The listing builds one solid part. Answer for the finished solid, in the listing's coordinates (mm). A direction names the side the tool comes from. Coordinates: 2 decimals unless noted, no trailing zeros. Order: outer loops, then holes, each group sorted by start corner. A loop starts at its lowest first (then second) coordinate and runs counter-clockwise, first axis right, second up. Notation, with made-up numbers: (-24.5, -2.75) - (-5.5, -2.75) arc R21 cw to (-5.5, 26.25) - close; hole circle Ø11 at (48.5, 71.25). An arc over 180 degrees is marked (long way). Use one line per item in the form item = value. Start each with the question number.
Item 1: The mould has two halves that part along X. Classify faces 1 (the flat face through (-52, 1.5, -61)), 2 (the cylindrical face through (-1.271, 0.021, -129.994)), 3 (the flat face through (48.734, 0.021, -39.41)), 4 (the flat face through (-50.12, 0.02, -41.06)): released by +X, released by -X, zero draft, split by the parting line, or undercut.
Item 2: Section A-A, the plane z = -65.5 is taken. Write down the section's boundary in (x, y).
Item 3: A tool of negligible diameter and unlimited length cuts with its end or side. For faces 5 (the flat face through (-52, -1.5, -61)), 6 (the flat face through (42.366, 0.021, -50.49)), from which of +Z, -Z, +X, -X, +Y, -Y can it reach the whole face along a straight path? Write none if from no direction.
Item 4: Section B-B, the plane x = 55 is taken. Write down the section's boundary in (y, z), and give its area (3 significant figures).
Item 5: Each of these flat-tipped pins is pushed along its axis until it touches: pin 1 Ø1 at (y, z) = (-1, -69.5) entering from +X; pin 2 Ø12 at (x, z) = (7.5, -14.5) entering from -Y; pin 3 Ø2.5 at (x, z) = (-20.65, -11.93) entering from +Y. Where does it stop, or does it pass through?
Item 6: Section C-C, the plane y = -0.3 is taken. Write down the section's boundary in (x, z), and give its area (3 significant figures).
Item 7: Consider line 1 along X through (y, z) = (-0.85, -12); line 2 along X through (y, z) = (-1.3, -15.5); line 3 along Z through (x, y) = (75, -0.9). Determine where each line is inside the solid, lowest interval first. Write a range as [from, to].
from build123d import *

# Parameters (mm, degrees)
DODANIE_WYCI_GNI_CIE1_DEPTH = 1.5
OTWORY_USTALAJ_CE_4_0MM1_D  = 4


with BuildPart() as part:
    # Szkic1 → Dodanie-wyciągnięcie1 (new, symmetric)
    with BuildSketch(Plane(origin=(0, 0, 0), x_dir=(1, 0, 0), z_dir=(0, 1, 0))):
        with BuildLine():
            Line((-98.851612767, 99.138078726), (0, -18.668685922))
            Line((0, -18.668685922), (98.851612767, 99.138078726))
            ThreePointArc((98.851612767, 99.138078726), (94.507932102, 103.28722462), (89.990265356, 107.246222037))
            ThreePointArc((89.990265356, 107.246222037), (0, 140), (-89.990265356, 107.246222037))
            ThreePointArc((-89.990265356, 107.246222037), (-94.507932102, 103.28722462), (-98.851612767, 99.138078726))
        make_face()
        with BuildLine():
            Line((0, 0), (-83.562389259, 99.585777605))
            ThreePointArc((-83.562389259, 99.585777605), (0, 130), (83.562389259, 99.585777605))
            Line((83.562389259, 99.585777605), (0, 0))
        make_face(mode=Mode.SUBTRACT)
    extrude(amount=DODANIE_WYCI_GNI_CIE1_DEPTH, both=True)

    # Otwory ustalające Ø4.0mm1 (through all)
    with Locations(Plane(origin=(0, 1.5, 0), x_dir=(1, 0, 0), z_dir=(0, 1, 0))):
        with Locations((65, 50), (-65, 50), (-20.649569124, 11.932485481)):
            Hole(OTWORY_USTALAJ_CE_4_0MM1_D / 2)


solid = part.part
Response:
q1.face_1 = zero draft
q1.face_2 = undercut
q1.face_3 = released by +X
q1.face_4 = released by -X
q2.outline = (-70.63, -1.5) - (-54.96, -1.5) - (-54.96, 1.5) - (-70.63, 1.5) - close; (54.96, -1.5) - (70.63, -1.5) - (70.63, 1.5) - (54.96, 1.5) - close
q3.face_5 = +Z, -Z, +X, -X, -Y
q3.face_6 = +Y, -Y
q4.outline = (-1.5, -128.74) - (1.5, -128.74) - (1.5, -117.79) - (-1.5, -117.79) - close; (-1.5, -65.55) - (1.5, -65.55) - (1.5, -46.88) - (-1.5, -46.88) - close
q4.area = 88.9 mm2
q5.pin_1 = 74.4
q5.pin_2 = -1.5
q5.pin_3 = through
q6.outline = (-98.85, -99.14) arc R140 ccw to (98.85, -99.14) - (0, 18.67) - close; hole (-83.56, -99.59) arc R130 ccw to (83.56, -99.59) - (0, 0) - close; hole circle Ø4 at (-20.65, -11.93)
q6.area = 5,400 mm2
q7.line_1 = [-25.73, -22.65], [-18.65, -10.07], [10.07, 25.73]
q7.line_2 = [-28.67, -13.01], [13.01, 28.67]
q7.line_3 = [-118.22, -106.18], [-89.38, -70.71]
